Verification items for the finished model (mm, model axes). Face numbers are marked on the shaded views. A direction names the side the tool comes from. Round coordinates to 2 decimals unless told otherwise and drop trailing zeros. Write each loop counter-clockwise with the first axis right and the second up, starting at its lowest first coordinate (ties: lowest second). Pieces come first, ordered by that corner, then holes. Notation, with made-up numbers: (38, 79) - (75, 79) arc R8 cw to (75, 89) - close; hole circle Ø4 at (41, -30). An arc over 180 degrees is marked (long way). Answer as a JSON object with one key per item and string values.
```python
from build123d import *

# Parameters (mm, degrees)
F0_R     = 12.7
F1_DEPTH = 6.35
F2_R     = 9.525
F3_DEPTH = 12.7
F4_R     = 12.7
F5_DEPTH = 6.35
F7_D     = 2.3876
F7_DEPTH = 3.175
F7_TIP   = 0.717307407
F9_D     = 12.7


with BuildPart() as f1:
    # F0 (on Front) → F1 (new body)
    with BuildSketch(Plane.XZ):
        Circle(F0_R)
    extrude(amount=F1_DEPTH)

    # F2 (on face) → F3 (join)
    with BuildSketch(Plane.XZ.offset(6.35)):
        Circle(F2_R)
    extrude(amount=F3_DEPTH)

    # F4 (on face) → F5 (join)
    with BuildSketch(Plane.XZ.offset(19.05)):
        Circle(F4_R)
    extrude(amount=F5_DEPTH)

    # F7
    with Locations(Plane.XZ.offset(25.4)):
        with Locations((-8.255, 0), (0, 8.255), (8.255, 0), (0, -8.255)):
            Hole(F7_D / 2, depth=F7_DEPTH)
            with Locations((0, 0, -(F7_DEPTH + F7_TIP / 2))):  # 118° drill point
                Cone(0, F7_D / 2, F7_TIP, mode=Mode.SUBTRACT)

    # F9 (through all)
    with Locations(Plane.XZ.offset(25.4)):
        with Locations((0, 0)):
            Hole(F9_D / 2)


solid = f1.part
```
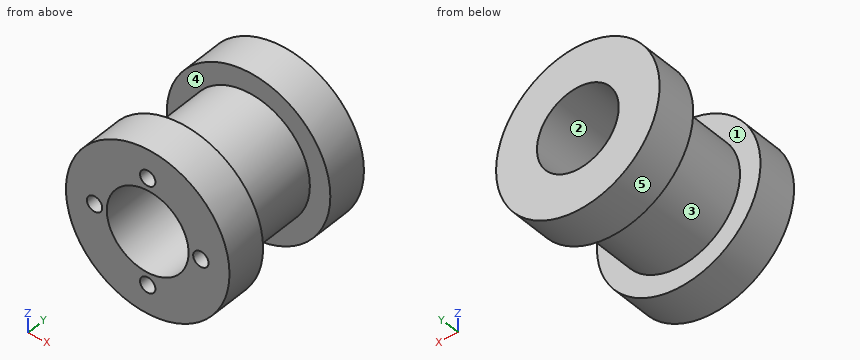
1. Cross-section at B-B (z = 2.25). Record the boundary of the cut face in (x, y).
Completed:
{"outline": "(-12.5, -25.4) - (-5.94, -25.4) - (-5.94, 0) - (-12.5, 0) - (-12.5, -6.35) - (-9.26, -6.35) - (-9.26, -19.05) - (-12.5, -19.05) - close; (5.94, -25.4) - (12.5, -25.4) - (12.5, -19.05) - (9.26, -19.05) - (9.26, -6.35) - (12.5, -6.35) - (12.5, 0) - (5.94, 0) - close"}
2. Cross-section at D-D (x = -10.5). Record the boundary of the cut face in (y, z), plus the area to 3 significant figures.
Completed:
{"outline": "(-25.4, -7.14) - (-19.05, -7.14) - (-19.05, 7.14) - (-25.4, 7.14) - close; (-6.35, -7.14) - (0, -7.14) - (0, 7.14) - (-6.35, 7.14) - close", "area": "181 mm^2"}
3. Cross-section at A-A (x = -5). Record the boundary of the cut face in (y, z).
Completed:
{"outline": "(-25.4, -11.67) - (-19.05, -11.67) - (-19.05, -8.11) - (-6.35, -8.11) - (-6.35, -11.67) - (0, -11.67) - (0, -3.91) - (-25.4, -3.91) - close; (-25.4, 3.91) - (0, 3.91) - (0, 11.67) - (-6.35, 11.67) - (-6.35, 8.11) - (-19.05, 8.11) - (-19.05, 11.67) - (-25.4, 11.67) - close"}
4. Go/stop test with flat-tipped pins: pin 1 (2 mm diameter, centred on x = 0, z = 8.255, fed in from -Y); pin 2 (3 mm diameter, centred on x = -9, y = -10.5, fed in from +Z); pin 3 (4 mm diameter, centred on x = 7, y = -21.5, fed in from +Z). Record where each tip stops, or that it passes through.
Completed:
{"pin 1": "stops at y = -22.11", "pin 2": "stops at z = 5.87", "pin 3": "stops at z = 11.67"}
5. Cross-section at C-C (y = -21). Record the boundary of the cut face in (x, z).
Completed:
{"outline": "circle Ø25.4 at (0, 0); hole circle Ø12.7 at (0, 0)"}
6. Mould release check, pull along Z, two halves, no side actions. Record for the marked faces 1, 2 and 3: released by +Z, released by -Z, zero draft, split by the parting line, or undercut.
Completed:
{"face 1": "zero draft", "face 2": "undercut", "face 3": "split by the parting line"}
7. Access from +Z, -Z, +X, -X, +Y, -Y to the whole of each face (thin tool, end or side, straight path). Record for the marked faces 4 and 5.
Completed:
{"face 4": "none", "face 5": "+Y, -Y"}
8. Material ranges on probe 1 along Z at (x, y) = (0, -24.15); probe 2 along Y at (x, z) = (10.75, 5.75); probe 3 along Z at (x, y) = (0, -19.75), recorded low to high. Write a range as from..to.
Completed:
{"probe 1": "z = -12.7..-9.45, -7.06..-6.35, 6.35..7.06, 9.45..12.7", "probe 2": "y = -25.4..-19.05, -6.35..0", "probe 3": "z = -12.7..-6.35, 6.35..12.7"}
